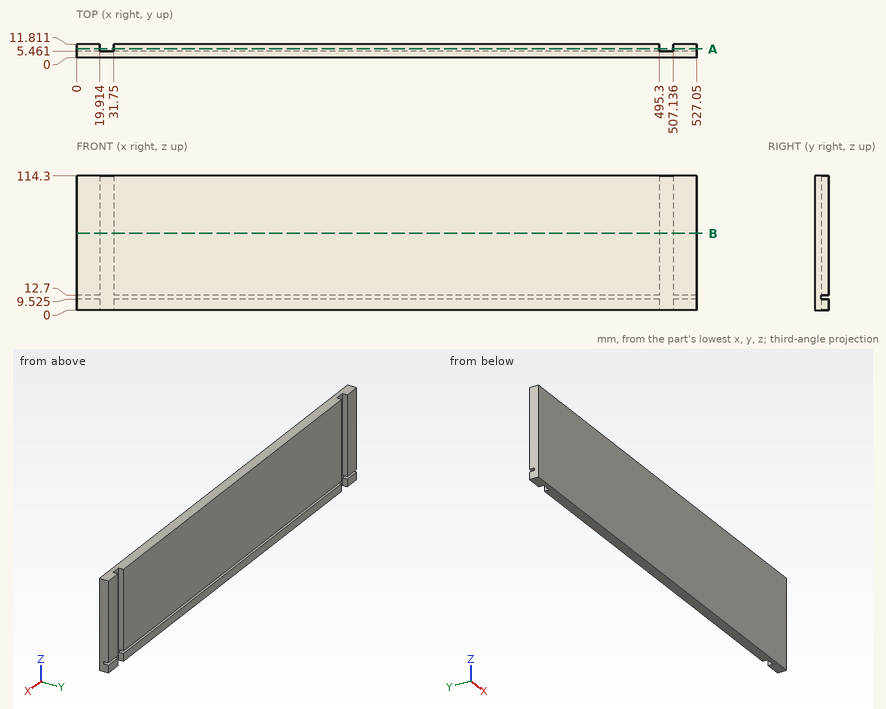
Input: dimensioned drawing with shaded views. Units: mm. Origin: part minimum x, y, z. Give positions to 0.01 mm unless a question says otherwise; leave off trailing zeros. Loops run counter-clockwise (first coordinate to the right, second up) from the corner with the lowest first, then second, coordinate; pieces in that order, holes last. Notation, with made-up numbers: M -29,-16 L 5,-16 A25 ccw 5,19 Z; hole C 5,-4.5 d2. An arc over 180 degrees is marked long. Put each result on its own line as item: value.
1) Cut plane B-B, the plane z = 65.5. Return the cut outline in (x, y).
Computed values:
outline: M 0,0 L 527.05,0 L 527.05,11.81 L 507.14,11.81 L 507.14,5.46 L 495.3,5.46 L 495.3,11.81 L 31.75,11.81 L 31.75,5.46 L 19.91,5.46 L 19.91,11.81 L 0,11.81 Z
2) Cut plane A-A, the plane y = 7.75. Give the number of separate pieces and of enclosed holes in the cut face, plus the area to 3 significant figures.
Computed values:
separate pieces: 6
enclosed holes: 0
area: 55,900 mm^2
3) Material intervals for L1, parallel to X at y = 5.75, z = 37; L2, parallel to Z at x = 227, y = 5.5 (1 decimal), sorted ascending. Write a range as from..to.
Computed values:
L1: x = 0..19.91, 31.75..495.3, 507.14..527.05
L2: z = 0..9.5, 12.7..114.3
